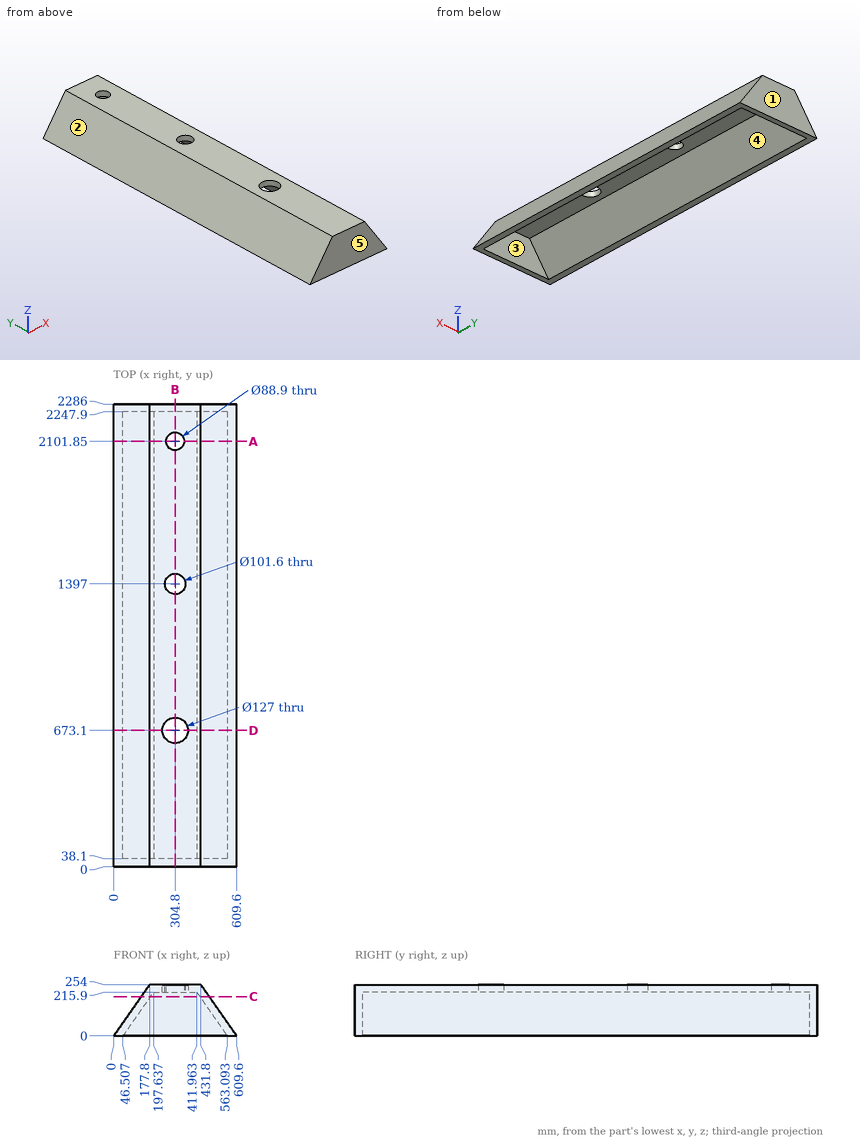
Design review of the part shown in the three views and the two pictorial views. Dimensions are in mm from the part's minimum x, y and z. A direction names the side the tool comes from. Give positions to 0.01 mm unless a question says otherwise; leave off trailing zeros. Loops run counter-clockwise (first coordinate to the right, second up) from the corner with the lowest first, then second, coordinate; pieces in that order, holes last. Notation, with made-up numbers: (77.25, 58.25) - (112.25, 58.25) arc R22 cw to (112.25, 72.25) - close; hole circle Ø5 at (70, 5). An arc over 180 degrees is marked (long way). Use CSV: the item, a comma, the result in double quotes. Start each with the question number.
1. Add section A-A (y = 2101.85). State the section outline as (x, z) points, plus the area to 3 significant figures.
2. Machinability: for the marked faces 4 and 5, which of the approach directions +Z, -Z, +X, -X, +Y, -Y give a long, thin tool a straight path to every point of the face, cutting with its end or side? Answer none if there is none.
3. Add section D-D (y = 673.1). State the section outline as (x, z) points, plus the area to 3 significant figures.
4. Draft analysis for pull direction X (two halves, no side actions). For the marked faces 1, 2 and 3, state which applies: released by +X, released by -X, zero draft, split by the parting line, or undercut.
5. Insertion check: P1, Ø4, axis at y = 1094.5, z = 157, coming from the +X side; P2, Ø6, axis at x = 447.5, y = 312.5, coming from the +Z side; P3, Ø2, axis at y = 1847, z = 93.5, coming from the +X side. Each pin has a flat end and moves straight along its axis. Give the tip position at first contact, or say it passes through.
6. Add section B-B (x = 304.8). State the section outline as (y, z) points.
7. Add section C-C (z = 195). State the section outline as (x, y) points.
8. Wall thickness on L1, parallel to Y at x = 304, z = 241 (3 decimals); L2, parallel to Y at x = 247.5, z = 66.5; L3, parallel to Z at x = 425, y = 333.5: over which ranges is each line inside the solid? List them lowest first.
Results found:
1,outline,"(0, 0) - (46.51, 0) - (197.64, 215.9) - (260.35, 215.9) - (260.35, 254) - (177.8, 254) - close; (349.25, 215.9) - (411.96, 215.9) - (563.09, 0) - (609.6, 0) - (431.8, 254) - (349.25, 254) - close"
1,area,"27,400 mm²"
2,face 4,"-Z"
2,face 5,"+Z, -Z, +X, -X, -Y"
3,outline,"(0, 0) - (46.51, 0) - (197.64, 215.9) - (241.3, 215.9) - (241.3, 254) - (177.8, 254) - close; (368.3, 215.9) - (411.96, 215.9) - (563.09, 0) - (609.6, 0) - (431.8, 254) - (368.3, 254) - close"
3,area,"25,900 mm²"
4,face 1,"zero draft"
4,face 2,"released by -X"
4,face 3,"undercut"
5,P1,"stops at x = 501.1"
5,P2,"stops at z = 235.86"
5,P3,"stops at x = 544.85"
6,outline,"(0, 0) - (38.1, 0) - (38.1, 215.9) - (609.6, 215.9) - (609.6, 254) - (0, 254) - close; (736.6, 215.9) - (1346.2, 215.9) - (1346.2, 254) - (736.6, 254) - close; (1447.8, 215.9) - (2057.4, 215.9) - (2057.4, 254) - (1447.8, 254) - close; (2146.3, 215.9) - (2247.9, 215.9) - (2247.9, 0) - (2286, 0) - (2286, 254) - (2146.3, 254) - close"
7,outline,"(136.5, 0) - (473.1, 0) - (473.1, 2286) - (136.5, 2286) - close; hole (183.01, 38.1) - (426.59, 38.1) - (426.59, 2247.9) - (183.01, 2247.9) - close"
8,L1,"y = 0 to 609.605, 736.595 to 1346.206, 1447.794 to 2057.407, 2146.293 to 2286"
8,L2,"y = 0 to 38.1, 2247.9 to 2286"
8,L3,"z = 197.28 to 254"
